```python
from build123d import *

# Parameters (mm, degrees)
SKETCH1_R           = 19.05
SKETCH1_R_2         = 1.375
SKETCH1_R_3         = 4.7625
BOSS_EXTRUDE1_DEPTH = 3.175
SKETCH2_R           = 11.43
CUT_EXTRUDE1_DEPTH  = 1.27


with BuildPart() as part:
    # Sketch1 → Boss-Extrude1 (new body)
    with BuildSketch(Plane.XY):
        Circle(SKETCH1_R)
        with Locations((0, 15.875)):
            Circle(SKETCH1_R_2, mode=Mode.SUBTRACT)
        with Locations((11.225320151, 11.225320151)):
            Circle(SKETCH1_R_2, mode=Mode.SUBTRACT)
        with Locations((15.875, 0)):
            Circle(SKETCH1_R_2, mode=Mode.SUBTRACT)
        Circle(SKETCH1_R_3, mode=Mode.SUBTRACT)
        with Locations((11.225320151, -11.225320151)):
            Circle(SKETCH1_R_2, mode=Mode.SUBTRACT)
        with Locations((0, -15.875)):
            Circle(SKETCH1_R_2, mode=Mode.SUBTRACT)
        with Locations((-11.225320151, -11.225320151)):
            Circle(SKETCH1_R_2, mode=Mode.SUBTRACT)
        with Locations((-15.875, 0)):
            Circle(SKETCH1_R_2, mode=Mode.SUBTRACT)
        with Locations((-11.225320151, 11.225320151)):
            Circle(SKETCH1_R_2, mode=Mode.SUBTRACT)
    extrude(amount=BOSS_EXTRUDE1_DEPTH)

    # Sketch2 → Cut-Extrude1 (cut)
    with BuildSketch(Plane.XY.offset(3.175)):
        Circle(SKETCH2_R)
    extrude(amount=-CUT_EXTRUDE1_DEPTH, mode=Mode.SUBTRACT)


solid = part.part
```
Work out the finished part from the listing and answer in its coordinate system (mm). A direction names the side the tool comes from. Round coordinates to 2 decimals unless told otherwise and drop trailing zeros. Write each loop counter-clockwise with the first axis right and the second up, starting at its lowest first coordinate (ties: lowest second). Pieces come first, ordered by that corner, then holes. Notation, with made-up numbers: (4, 69.25) -> (53, 69.25) arc R13 ccw to (53, 78.25) -> close; hole circle Ø8 at (-12.5, 68.5). An arc over 180 degrees is marked (long way). Write each question's results on one line, items separated by ' | '.
1) The part is cut by section D-D (x = 10.5). Write down the section's boundary in (y, z) (3 decimals), and give its area (3 significant figures).
Findings:
outline: (-15.895, 0) -> (-12.393, 0) -> (-12.393, 3.175) -> (-15.895, 3.175) -> close; (-10.057, 0) -> (10.057, 0) -> (10.057, 3.175) -> (4.516, 3.175) -> (4.516, 1.905) -> (-4.516, 1.905) -> (-4.516, 3.175) -> (-10.057, 3.175) -> close; (12.393, 0) -> (15.895, 0) -> (15.895, 3.175) -> (12.393, 3.175) -> close | area: 74.6 mm²
2) The part is cut by section C-C (y = -15). Write down the section's boundary in (x, z) (3 decimals), and give its area (3 significant figures).
Findings:
outline: (-11.743, 0) -> (-1.061, 0) -> (-1.061, 3.175) -> (-11.743, 3.175) -> close; (1.061, 0) -> (11.743, 0) -> (11.743, 3.175) -> (1.061, 3.175) -> close | area: 67.8 mm²
3) For a pull along X with two mould halves and no side action, classify faces 1 (the flat face through (4, -4, 0)), 2 (the cylindrical face through (-3.78, -2.9, 0.94)), 3 (the cylindrical face through (-15.12, -11.59, 1.57)) as +X half, -X half, draft (parallel to the pull), parting line (faces both ways), or undercut.
Findings:
face 1: draft | face 2: undercut | face 3: parting line
4) Flat-ended cylindrical pins translate along their axes: pin 1 (5 mm diameter, centred on x = 14, y = 1, fed in from -Z); pin 2 (2 mm diameter, centred on x = -11.23, y = -11.23, fed in from -Z); pin 3 (7 mm diameter, centred on x = -5.5, y = -5.5, fed in from +Z) (3 decimals). Find the tip coordinate at first contact, or state that the pin passes through.
Findings:
pin 1: stops at z = 0 | pin 2: passes through | pin 3: stops at z = 1.905
5) Consider line 1 along Y through (x, z) = (0, 1.2); line 2 along Y through (x, z) = (0, 2); line 3 along X through (y, z) = (-12, 2). Determine where each line is inside the solid, lowest interval first. Write a range as [from, to].
Findings:
line 1: y = [-19.05, -17.25], [-14.5, -4.76], [4.76, 14.5], [17.25, 19.05] | line 2: y = [-19.05, -17.25], [-14.5, -11.43], [11.43, 14.5], [17.25, 19.05] | line 3: x = [-14.8, -12.36], [-10.09, 10.09], [12.36, 14.8]
6) Which of the six approach directions +Z, -Z, +X, -X, +Y, -Y give full straight-line access (tool end or side, diameter ignored) to faces 4 (the cylindrical face through (10.902, 3.433, 2.549)), 5 (the cylindrical face through (10.21, 12.15, 1.57))?
Findings:
face 4: +Z | face 5: +Z, -Z
7) The part is cut by section A-A (y = 0). State how many separate pieces and enclosed holes the cut face has, and give its area (3 significant figures).
Findings:
separate pieces: 4 | enclosed holes: 0 | area: 56.3 mm²
